Geometry: see drawing. Coordinates: mm, zero at the bounding-box minimum. A direction names the side the tool comes from. Round coordinates to 2 decimals unless told otherwise and drop trailing zeros. Write each loop counter-clockwise with the first axis right and the second up, starting at its lowest first coordinate (ties: lowest second). Pieces come first, ordered by that corner, then holes. Notation, with made-up numbers: M 5,36.25 L 60,36.25 A24 cw 60,57.25 Z; hole C 80.25,17.5 d7. An arc over 180 degrees is marked long. Use one line per item in the form item = value. Start each with the question number.
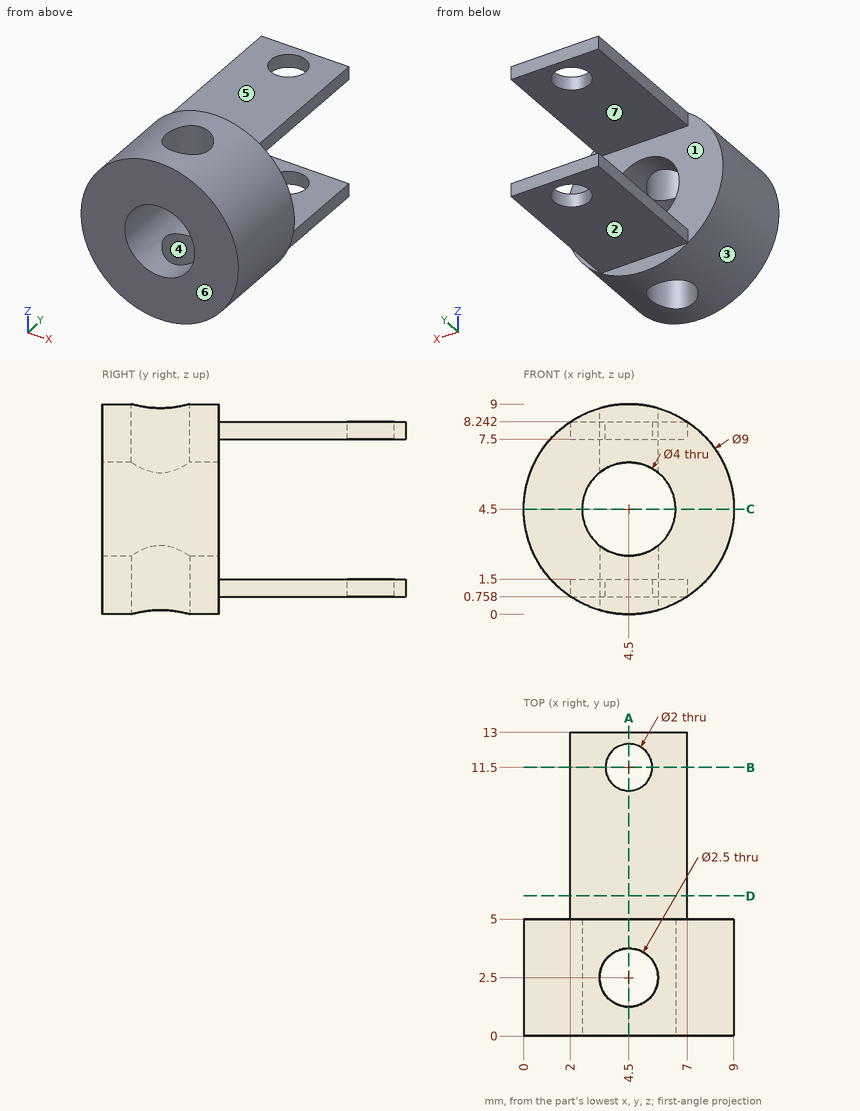
Item 1: Draft query along Z for the marked faces 1, 2, 3 and 4. Return one class per face: +Z half, -Z half, draft (parallel to the pull), parting line (faces both ways), or undercut.
Item 2: Cut plane A-A (x = 4.5). Give the number of separate pieces and of enclosed holes in the cut face, plus the area to 3 significant figures.
Item 3: Ray query, line 1 (Z direction, x = 4, y = 8); line 2 (X direction, y = 1, z = 2); line 3 (Y direction, x = 1, z = 7.25). Return the intervals inside material, ascending. Write a range as from..to.
Item 4: First-contact query: pin 1 (2 mm diameter, centred on x = 6.5, z = 3.5, fed in from +Y); pin 2 (1 mm diameter, centred on x = 7, y = 5, fed in from -Z); pin 3 (0.6 mm diameter, centred on y = 7.5, z = 1, fed in from -X). Flat tips, straight axial feed; report the tip coordinate or a pass-through.
Item 5: Cut plane D-D (y = 6). Output: boundary loops of the cut face in (x, z).
Item 6: Reachability of the marked faces 5, 6 and 7 from +Z, -Z, +X, -X, +Y, -Y: full face, straight path, thin tool, end or side. Return the list, or none.
Item 7: Cut plane C-C (z = 4.5). Output: boundary loops of the cut face in (x, y), plus the area to 3 significant figures.
Item 8: Cut plane B-B (y = 11.5). Output: boundary loops of the cut face in (x, z).
Final values:
q1.face_1 = undercut
q1.face_2 = -Z half
q1.face_3 = parting line
q1.face_4 = draft
q2.separate_pieces = 6
q2.enclosed_holes = 0
q2.area = 21.4 mm^2
q3.line_1 = 0.76..1.5, 7.5..8.24
q3.line_2 = 0.76..8.24
q3.line_3 = 0..5
q4.pin_1 = 5
q4.pin_2 = 0.47
q4.pin_3 = 2
q5.outline = M 2,0.76 L 7,0.76 L 7,1.5 L 2,1.5 Z; M 2,7.5 L 7,7.5 L 7,8.24 L 2,8.24 Z
q6.face_5 = +Z, +X, -X, +Y
q6.face_6 = +Z, -Z, +X, -X, -Y
q6.face_7 = +X, -X, +Y
q7.outline = M 0,0 L 2.5,0 L 2.5,5 L 0,5 Z; M 6.5,0 L 9,0 L 9,5 L 6.5,5 Z
q7.area = 25.0 mm^2
q8.outline = M 2,0.76 L 3.5,0.76 L 3.5,1.5 L 2,1.5 Z; M 2,7.5 L 3.5,7.5 L 3.5,8.24 L 2,8.24 Z; M 5.5,0.76 L 7,0.76 L 7,1.5 L 5.5,1.5 Z; M 5.5,7.5 L 7,7.5 L 7,8.24 L 5.5,8.24 Z
